For this review, take the finished solid that the model builds, in its own axes (mm). A direction names the side the tool comes from. Coordinates: 2 decimals unless noted, no trailing zeros. Loops run counter-clockwise (first coordinate to the right, second up) from the corner with the lowest first, then second, coordinate; pieces in that order, holes last. Notation, with made-up numbers: M 19.25,36 L 55.25,36 A18 cw 55.25,71 Z; hole C -11.5,-32 d10. An arc over 180 degrees is marked long. Use one line per item in the form item = value.
```python
from build123d import *

# Parameters (mm, degrees)
F1_DEPTH = 88.9
F3_DEPTH = 88.901
F4_SCALE = 0.0114810563


with BuildPart() as f1:
    # F0 (on Right) → F1 (new body)
    with BuildSketch(Plane.YZ):
        Polygon((0, 3048), (0, 0), (3048, 0), (3048, 4267.2), align=None)
    extrude(amount=F1_DEPTH)

    # F2 (on face) → F3 (cut, through all)
    with BuildSketch(Plane.YZ.offset(88.9)):
        Polygon((406.4, 3169.5250441696), (38.1, 3022.2050441696), (38.1, 38.1), (406.4, 38.1), align=None)
        Polygon((812.8, 3332.0850441696), (444.5, 3184.7650441696), (444.5, 38.1), (812.8, 38.1), align=None)
        Polygon((1219.2, 3494.6450441696), (850.9, 3347.3250441696), (850.9, 38.1), (1219.2, 38.1), align=None)
        Polygon((1625.6, 3657.2050441696), (1257.3, 3509.8850441696), (1257.3, 38.1), (1625.6, 38.1), align=None)
        Polygon((2032, 3819.7650441696), (1663.7, 3672.4450441696), (1663.7, 38.1), (2032, 38.1), align=None)
        Polygon((2438.4, 3982.3250441696), (2070.1, 3835.0050441696), (2070.1, 38.1), (2438.4, 38.1), align=None)
        Polygon((2844.8, 4144.8850441696), (2476.5, 3997.5650441696), (2476.5, 38.1), (2844.8, 38.1), align=None)
        Polygon((3009.9, 4210.9250441696), (2882.9, 4160.1250441696), (2882.9, 38.1), (3009.9, 38.1), align=None)
    extrude(amount=-F3_DEPTH, mode=Mode.SUBTRACT)


with BuildPart() as f1_1:
    # F4: moved
    add(f1.part.scale(F4_SCALE))


solid = f1_1.part
```
1. Consider section A-A on z = 41.5. Write out the cut boundary in (x, y).
Computed values:
outline = M 0,16.26 L 1.02,16.26 L 1.02,17.44 L 0,17.44 Z; M 0,18.66 L 1.02,18.66 L 1.02,19.1 L 0,19.1 Z; M 0,23.33 L 1.02,23.33 L 1.02,23.77 L 0,23.77 Z; M 0,28 L 1.02,28 L 1.02,28.43 L 0,28.43 Z; M 0,32.66 L 1.02,32.66 L 1.02,33.1 L 0,33.1 Z; M 0,34.56 L 1.02,34.56 L 1.02,34.99 L 0,34.99 Z
2. Consider section C-C on z = 30. State how many separate pieces and enclosed holes the cut face has, plus the area to 3 significant figures.
Computed values:
separate_pieces = 9
enclosed_holes = 0
area = 4.02 mm2
3. Draft analysis for pull direction Y (two halves, no side actions). For faces 1 (the face through (0.5, 0, 17.7)), 2 (the face through (0.5, 27.995, 22.8)), state which applies: +Y half, -Y half, draft (parallel to the pull), parting line (faces both ways), or undercut.
Computed values:
face_1 = -Y half
face_2 = undercut
4. Wall thickness on line 1 along Z through (x, y) = (0.9, 7.5); line 2 along Z through (x, y) = (0.4, 16.5); line 3 along Z through (x, y) = (0.6, 9.5): over which ranges is each line inside the solid? List them lowest first. Write a range as from..to.
Computed values:
line_1 = 0..0.44, 37.52..37.99
line_2 = 0..0.44, 41.12..41.59
line_3 = 0..38.79
5. Consider section B-B on y = 25.5. Write out the cut boundary in (x, z), plus the area to 3 significant figures.
Computed values:
outline = M 0,0 L 1.02,0 L 1.02,0.44 L 0,0.44 Z; M 0,44.72 L 1.02,44.72 L 1.02,45.19 L 0,45.19 Z
area = 0.927 mm2
6. Tool access review of faces 3 (the face through (0.5, 17.74, 42.09)), 4 (the face through (0.5, 13.998, 20)): name each direction out of +Z, -Z, +X, -X, +Y, -Y from which nothing blocks a thin tool from reaching the whole face with its end or side.
Computed values:
face_3 = +Z, +X, -X, -Y
face_4 = +X, -X
